from build123d import *

# Parameters (mm, degrees)
PAD_DEPTH      = 150
SKETCH_R       = 1.7
HOLE_DEPTH     = 25
HOLE_TIPS_R    = 1.7
SKETCH008_R    = 1.7
HOLE001_DEPTH  = 25
HOLE001_TIPS_R = 1.7
SKETCH009_R    = 1.7
HOLE002_DEPTH  = 25
HOLE002_TIPS_R = 1.7
SKETCH010_W    = 60
SKETCH010_H    = 120
PAD001_DEPTH   = 12
SKETCH012_W    = 60
SKETCH012_H    = 120
PAD002_DEPTH   = 12
SKETCH013_W    = 60
SKETCH013_H    = 120
PAD003_DEPTH   = 12
SKETCH015_W    = 60
SKETCH015_H    = 120
PAD004_DEPTH   = 12
SKETCH016_W    = 60
SKETCH016_H    = 120
PAD005_DEPTH   = 12
SKETCH017_W    = 60
SKETCH017_H    = 120
PAD006_DEPTH   = 12


with BuildPart() as part:
    # Sketch007 → Pad (new body)
    with BuildSketch(Plane.XY):
        Polygon((88.334591186, 51), (0, 102), (-88.334591186, 51), (-88.334591186, -51), (0, -102), (88.334591186, -51), align=None)
        Polygon((86.6025403784, 50), (0, 100), (-86.6025403784, 50), (-86.6025403784, -50), (0, -100), (86.6025403784, -50), align=None, mode=Mode.SUBTRACT)
    extrude(amount=PAD_DEPTH)

    # Sketch (on Face6 of Pad) → Hole (cut)
    with BuildSketch(Plane.YZ.offset(88.334591186)):
        with Locations((0, 5)):
            Circle(SKETCH_R)
        with Locations((0, 145)):
            Circle(SKETCH_R)
    extrude(amount=-HOLE_DEPTH, mode=Mode.SUBTRACT)

    # Hole tips → Hole tip 1 section 0
    with BuildSketch(Plane.YZ.offset(63.334591186), mode=Mode.PRIVATE) as hole_tip_1_s0:
        with Locations((0, 5)):
            Circle(HOLE_TIPS_R)
    loft([hole_tip_1_s0.sketch, Vertex(62.3131281337, 0, 5)], mode=Mode.SUBTRACT)

    # Hole tips → Hole tip 2 section 0
    with BuildSketch(Plane.YZ.offset(63.334591186), mode=Mode.PRIVATE) as hole_tip_2_s0:
        with Locations((0, 145)):
            Circle(HOLE_TIPS_R)
    loft([hole_tip_2_s0.sketch, Vertex(62.3131281337, 0, 145)], mode=Mode.SUBTRACT)

    # Sketch008 (on Face3 of Hole) → Hole001 (cut)
    with BuildSketch(Plane(origin=(-44.167295593, 76.5, 0), x_dir=(-0.8660254038, -0.5, 0), z_dir=(-0.5, 0.8660254038, 0))):
        with Locations((0, 5)):
            Circle(SKETCH008_R)
        with Locations((0, 145)):
            Circle(SKETCH008_R)
    extrude(amount=-HOLE001_DEPTH, mode=Mode.SUBTRACT)

    # Hole001 tips → Hole001 tip 1 section 0
    with BuildSketch(Plane(origin=(-31.667295593, 54.8493649054, 0), x_dir=(-0.8660254038, -0.5, 0), z_dir=(-0.5, 0.8660254038, 0)), mode=Mode.PRIVATE) as hole001_tip_1_s0:
        with Locations((0, 5)):
            Circle(HOLE001_TIPS_R)
    loft([hole001_tip_1_s0.sketch, Vertex(-31.1565640668, 53.964751953, 5)], mode=Mode.SUBTRACT)

    # Hole001 tips → Hole001 tip 2 section 0
    with BuildSketch(Plane(origin=(-31.667295593, 54.8493649054, 0), x_dir=(-0.8660254038, -0.5, 0), z_dir=(-0.5, 0.8660254038, 0)), mode=Mode.PRIVATE) as hole001_tip_2_s0:
        with Locations((0, 145)):
            Circle(HOLE001_TIPS_R)
    loft([hole001_tip_2_s0.sketch, Vertex(-31.1565640668, 53.964751953, 145)], mode=Mode.SUBTRACT)

    # Sketch009 (on Face10 of Hole) → Hole002 (cut)
    with BuildSketch(Plane(origin=(-44.167295593, -76.5, 0), x_dir=(0.8660254038, -0.5, 0), z_dir=(-0.5, -0.8660254038, 0))):
        with Locations((0, 5)):
            Circle(SKETCH009_R)
        with Locations((0, 145)):
            Circle(SKETCH009_R)
    extrude(amount=-HOLE002_DEPTH, mode=Mode.SUBTRACT)

    # Hole002 tips → Hole002 tip 1 section 0
    with BuildSketch(Plane(origin=(-31.667295593, -54.8493649054, 0), x_dir=(0.8660254038, -0.5, 0), z_dir=(-0.5, -0.8660254038, 0)), mode=Mode.PRIVATE) as hole002_tip_1_s0:
        with Locations((0, 5)):
            Circle(HOLE002_TIPS_R)
    loft([hole002_tip_1_s0.sketch, Vertex(-31.1565640668, -53.964751953, 5)], mode=Mode.SUBTRACT)

    # Hole002 tips → Hole002 tip 2 section 0
    with BuildSketch(Plane(origin=(-31.667295593, -54.8493649054, 0), x_dir=(0.8660254038, -0.5, 0), z_dir=(-0.5, -0.8660254038, 0)), mode=Mode.PRIVATE) as hole002_tip_2_s0:
        with Locations((0, 145)):
            Circle(HOLE002_TIPS_R)
    loft([hole002_tip_2_s0.sketch, Vertex(-31.1565640668, -53.964751953, 145)], mode=Mode.SUBTRACT)

    # Sketch010 (on Face12 of Hole002) → Pad001 (join)
    with BuildSketch(Plane(origin=(-44.167295593, -76.5, 0), x_dir=(0.8660254038, -0.5, 0), z_dir=(-0.5, -0.8660254038, 0))):
        with Locations((0, 75)):
            Rectangle(SKETCH010_W, SKETCH010_H)
    extrude(amount=PAD001_DEPTH)

    # Sketch012 (on Face6 of Hole002) → Pad002 (join)
    with BuildSketch(Plane(origin=(44.167295593, -76.5, 0), x_dir=(0.8660254038, 0.5, 0), z_dir=(0.5, -0.8660254038, 0))):
        with Locations((0, 75)):
            Rectangle(SKETCH012_W, SKETCH012_H)
    extrude(amount=PAD002_DEPTH)

    # Sketch013 (on Face2 of Hole002) → Pad003 (join)
    with BuildSketch(Plane.YZ.offset(88.334591186)):
        with Locations((0, 75)):
            Rectangle(SKETCH013_W, SKETCH013_H)
    extrude(amount=PAD003_DEPTH)

    # Sketch015 (on Face1 of Hole002) → Pad004 (join)
    with BuildSketch(Plane(origin=(44.167295593, 76.5, 0), x_dir=(-0.8660254038, 0.5, 0), z_dir=(0.5, 0.8660254038, 0))):
        with Locations((0, 75)):
            Rectangle(SKETCH015_W, SKETCH015_H)
    extrude(amount=PAD004_DEPTH)

    # Sketch016 (on Face3 of Hole002) → Pad005 (join)
    with BuildSketch(Plane(origin=(-44.167295593, 76.5, 0), x_dir=(-0.8660254038, -0.5, 0), z_dir=(-0.5, 0.8660254038, 0))):
        with Locations((0, 75)):
            Rectangle(SKETCH016_W, SKETCH016_H)
    extrude(amount=PAD005_DEPTH)

    # Sketch017 (on Face9 of Hole002) → Pad006 (join)
    with BuildSketch(Plane(origin=(-88.334591186, 0, 0), x_dir=(0, -1, 0), z_dir=(-1, 0, 0))):
        with Locations((0, 75)):
            Rectangle(SKETCH017_W, SKETCH017_H)
    extrude(amount=PAD006_DEPTH)


solid = part.part
The model under review builds one solid part; all positions refer to its coordinate system, in mm. A direction names the side the tool comes from. Round coordinates to 2 decimals unless told otherwise and drop trailing zeros. Order: outer loops, then holes, each group sorted by start corner. A loop starts at its lowest first (then second) coordinate and runs counter-clockwise, first axis right, second up. Notation, with made-up numbers: (13.25, 5.25) -> (28.25, 5.25) arc R12 ccw to (28.25, 24.25) -> close; hole circle Ø11 at (89.25, 70). An arc over 180 degrees is marked (long way). Return JSON: item names as keys, results as strings.
1. For faces 5 (the face through (47, -82, 15)), 6 (the face through (-43.91, -74.65, 73.95)), 7 (the face through (47, 81, 135)), list the 3-axis set-ups (+Z, -Z, +X, -X, +Y, -Y) from which the entire face can be reached by the end or side of a thin tool; tool diameter is ignored.
Answer block:
{"face 5": "-Z, +X, -Y", "face 6": "+Z, -Z", "face 7": "+Z, +X, +Y"}
2. Take a section at A-A (y = 39.5). Write out the cut boundary in (x, z), then the cut area to 3 significant figures.
Answer block:
{"outline": "(-88.33, 0) -> (-86.6, 0) -> (-86.6, 150) -> (-88.33, 150) -> close; (86.6, 0) -> (88.33, 0) -> (88.33, 150) -> (86.6, 150) -> close", "area": "520 mm²"}
3. For L1, parallel to Z at x = 87, y = 0; L2, parallel to X at y = -39, z = 32.5; L3, parallel to X at y = 19, z = 82.5, list the stretches that pass through material, from the lowest coordinate up. Write a range as [from, to].
Answer block:
{"L1": "z = [0, 3.3], [6.7, 143.3], [146.7, 150]", "L2": "x = [-88.33, -86.6], [86.6, 88.33]", "L3": "x = [-100.33, -86.6], [86.6, 100.33]"}
4. Insertion check: P1, Ø3.5, axis at x = 92, y = 11.5, coming from the +Z side; P2, Ø8, axis at y = 56.5, z = 110.5, coming from the -X side; P3, Ø3, axis at x = 47, z = 59.5, coming from the -Y side. Each pin has a flat end and moves straight along its axis. Give the tip position at first contact, or say it passes through.
Answer block:
{"P1": "stops at z = 135", "P2": "stops at x = -85.74", "P3": "stops at y = -89.59"}
5. Take a section at B-B (x = 11). Write out the cut boundary in (y, z).
Answer block:
{"outline": "(-95.65, 0) -> (-93.65, 0) -> (-93.65, 150) -> (-95.65, 150) -> close; (93.65, 0) -> (95.65, 0) -> (95.65, 150) -> (93.65, 150) -> close"}
6. Take a section at C-C (y = -9.5). Write out the cut boundary in (x, z), then the cut area to 3 significant figures.
Answer block:
{"outline": "(-100.33, 15) -> (-88.33, 15) -> (-88.33, 0) -> (-86.6, 0) -> (-86.6, 150) -> (-88.33, 150) -> (-88.33, 135) -> (-100.33, 135) -> close; (86.6, 0) -> (88.33, 0) -> (88.33, 15) -> (100.33, 15) -> (100.33, 135) -> (88.33, 135) -> (88.33, 150) -> (86.6, 150) -> close", "area": "3,400 mm²"}
7. The part is to be moulded in two halves that separate along Y. For faces 1 (the face through (-73.106, -66.623, 74.16)), 2 (the face through (86.603, -1, 74)), 3 (the face through (-49.804, 87.102, 75.84)), 4 (the face through (-47, -81, 135)), say which applies: +Y half, -Y half, draft (parallel to the pull), parting line (faces both ways), or undercut.
Answer block:
{"face 1": "undercut", "face 2": "undercut", "face 3": "+Y half", "face 4": "draft"}
